Autodesk Fusion 360 part; units mm, degrees
sketch "Sketch5" plane through (0, 0, 4) normal (0, 0, 1) x (-1, 0, 0)
  arc A0 (84, -50) -> (88, -46) centre (84, -46) ccw
  line L0 (88, -46) -> (88, 46)
  arc A1 (88, 46) -> (84, 50) centre (84, 46) ccw
  line L1 (84, 50) -> (-84, 50)
  arc A2 (-84, 50) -> (-88, 46) centre (-84, 46) ccw
  line L2 (-88, 46) -> (-88, -46)
  arc A3 (-88, -46) -> (-84, -50) centre (-84, -46) ccw
  line L3 (-84, -50) -> (84, -50)
  circle A4 centre (69, -43.25) radius 1.425
  circle A5 centre (-69, -43.25) radius 7.5
  circle A6 centre (69, 43.25) radius 7.5
  circle A7 centre (-69, 43.25) radius 7.5
  circle A8 centre (69, -43.25) radius 3.5
  circle A9 centre (-69, -43.25) radius 2.5
  circle A10 centre (-69, 43.25) radius 2.5
  circle A11 centre (69, 43.25) radius 2.5
  line L4 (69, -43.25) -> (-69, -43.25) construction
  line L5 (69, -43.25) -> (69, 43.25) construction
  line L6 (85, -50) -> (85, -42.0241)
  line L7 (85, -42.0241) -> (85, 50) construction
  line L8 (-85, -50) -> (-85, 50) construction
  line L9 (0, -50) -> (0, 50) construction
  circle A12 centre (85, -35) radius 2.25
  circle A13 centre (85, 35) radius 1.425
  circle A14 centre (-85, -35) radius 1.425
  circle A15 centre (-85, 35) radius 1.425
  line L10 (88, 0) -> (-88, 0) construction
  line L11 (85, -35) -> (-85, -35) construction
  line L12 (85, 35) -> (-85, 35) construction
  line L13 (85, -32.75) -> (80, -32.75)
  arc A16 (80, -32.75) -> (80, -37.25) centre (80, -35) ccw
  line L14 (80, -37.25) -> (85, -37.25)
  arc A17 (85, -37.25) -> (85, -32.75) centre (85, -35) ccw
  line L15 (85, -35) -> (80, -35) construction
  line L16 (85, 37.25) -> (80, 37.25)
  arc A18 (80, 37.25) -> (80, 32.75) centre (80, 35) ccw
  line L17 (80, 32.75) -> (85, 32.75)
  arc A19 (85, 32.75) -> (85, 37.25) centre (85, 35) ccw
  line L18 (85, 35) -> (80, 35) construction
  line L19 (-85, -37.25) -> (-80, -37.25)
  arc A20 (-80, -37.25) -> (-80, -32.75) centre (-80, -35) ccw
  line L20 (-80, -32.75) -> (-85, -32.75)
  arc A21 (-85, -32.75) -> (-85, -37.25) centre (-85, -35) ccw
  line L21 (-85, -35) -> (-80, -35) construction
  line L22 (-85, 32.75) -> (-80, 32.75)
  arc A22 (-80, 32.75) -> (-80, 37.25) centre (-80, 35) ccw
  line L23 (-80, 37.25) -> (-85, 37.25)
  arc A23 (-85, 37.25) -> (-85, 32.75) centre (-85, 35) ccw
  line L24 (-85, 35) -> (-80, 35) construction
  point P0 (0, -43.25)
  point P1 (69, 0)
  dimension "d1" = 2.85
  dimension "d2" = 15
  dimension "d3" = 15
  dimension "d4" = 15
  dimension "d5" = 7
  dimension "d6" = 5
  dimension "d7" = 5
  dimension "d8" = 5
  dimension "d9" = 138
  dimension "d10" = 86.5
  dimension "d11" = 4.5
  dimension "d12" = 2.85
  dimension "d13" = 2.85
  dimension "d14" = 2.85
  dimension "d15" = 70
  dimension "d16" = 15
  dimension "d17" = 170
  dimension "d18" = 4.5
  dimension "d19" = 4.5
  dimension "d20" = 5
  dimension "d21" = 4.5
  dimension "d22" = 5
  dimension "d23" = 4.5
sketch "Sketch6" plane through (0, 0, 4) normal (0, 0, 1) x (-1, 0, 0)
  circle A0 centre (85, 35) radius 2.25
  circle A1 centre (-85, 35) radius 2.25
  circle A2 centre (85, -35) radius 2.25
  circle A3 centre (-85, -35) radius 2.25
  arc A4 (-88, -46) -> (-84, -50) centre (-84, -46) ccw
  line L0 (-84, -50) -> (84, -50)
  arc A5 (84, -50) -> (88, -46) centre (84, -46) ccw
  line L1 (88, -46) -> (88, 46)
  arc A6 (88, 46) -> (84, 50) centre (84, 46) ccw
  line L2 (84, 50) -> (-84, 50)
  arc A7 (-84, 50) -> (-88, 46) centre (-84, 46) ccw
  line L3 (-88, 46) -> (-88, -46)
  line L4 (32.925, -38.05) -> (-68.925, -38.05) construction
  line L5 (-68.925, -38.05) -> (-68.925, 38.05) construction
  line L6 (-68.925, 38.05) -> (32.925, 38.05) construction
  line L7 (32.925, 38.05) -> (32.925, -38.05) construction
  circle A8 centre (32.925, -38.05) radius 1.425
  circle A9 centre (32.925, -38.05) radius 3
  circle A10 centre (-68.925, -38.05) radius 1.425
  circle A11 centre (-68.925, -38.05) radius 3
  circle A12 centre (32.925, 38.05) radius 1.425
  circle A13 centre (32.925, 38.05) radius 3
  circle A14 centre (-68.925, 38.05) radius 1.425
  circle A15 centre (-68.925, 38.05) radius 3
  line L8 (22.8962, -40.5575) -> (-22.2991, -40.5575) construction
  line L9 (-22.2991, -40.5575) -> (-22.2991, -50.5575) construction
  line L10 (-22.2991, -50.5575) -> (22.8962, -50.5575) construction
  line L11 (22.8962, -50.5575) -> (22.8962, -40.5575) construction
  line L12 (32.925, -38.05) -> (-68.925, 38.05) construction
  line L13 (-68.925, -38.05) -> (32.925, 38.05) construction
  line L14 (28.925, -30.0681) -> (28.925, 30.0681)
  line L15 (28.925, 30.0681) -> (-11.3172, 0)
  line L16 (-11.3172, 0) -> (28.925, -30.0681)
  line L17 (20.8887, -34.05) -> (-18, -4.9932)
  line L18 (-18, -4.9932) -> (-56.8887, -34.05)
  line L19 (-56.8887, -34.05) -> (20.8887, -34.05)
  line L20 (-64.925, -30.0681) -> (-24.6828, 0)
  line L21 (-24.6828, 0) -> (-64.925, 30.0681)
  line L22 (-64.925, 30.0681) -> (-64.925, -30.0681)
  line L23 (-18, 4.9932) -> (20.8887, 34.05)
  line L24 (20.8887, 34.05) -> (-56.8887, 34.05)
  line L25 (-56.8887, 34.05) -> (-18, 4.9932)
  point P0 (32.925, 0)
  point P1 (0, -38.05)
  point P2 (0, -50)
  point P3 (-18, -38.05)
  dimension "d24" = 101.85
  dimension "d25" = 76.1
  dimension "d26" = 2.85
  dimension "d27" = 2.85
  dimension "d28" = 2.85
  dimension "d29" = 2.85
  dimension "d30" = 6
  dimension "d31" = 6
  dimension "d32" = 6
  dimension "d33" = 6
  dimension "d34" = 4
  dimension "d35" = 4
  dimension "d36" = 4
  dimension "d37" = 4
  dimension "d38" = 4
  dimension "d39" = 4
  dimension "d40" = 4
  dimension "d41" = 4
  dimension "d42" = 70
  dimension "d43" = 88
sketch "Sketch1" plane through (0, 0, 0) normal (0, 0, 1) x (1, 0, 0)
  line L0 (-88, 50) -> (88, 50)
  line L1 (88, 50) -> (88, -50)
  line L2 (88, -50) -> (-88, -50)
  line L3 (-88, -50) -> (-88, 50)
  point P0 (0, 50)
  point P1 (-88, 0)
  dimension "d57" = 176
  dimension "d58" = 100
extrude "Extrude1" add sketch "Sketch1" along normal blind 4
fillet "Fillet2" radius 4 4 edges at (-88, -50, 2) (-88, 50, 2) (88, -50, 2) (88, 50, 2)
extrude "Extrude5" cut sketch "Sketch5" against normal through all contours A12 A17 | A13 | A14 | A15
sketch "Sketch3" plane through (0, 0, 0) normal (0, 0, -1) x (1, 0, 0)
  arc A0 (84, -50) -> (88, -46) centre (84, -46) ccw
  line L0 (88, -46) -> (88, 46)
  arc A1 (88, 46) -> (84, 50) centre (84, 46) ccw
  line L1 (84, 50) -> (-84, 50)
  arc A2 (-84, 50) -> (-88, 46) centre (-84, 46) ccw
  line L2 (-88, 46) -> (-88, -46)
  arc A3 (-88, -46) -> (-84, -50) centre (-84, -46) ccw
  line L3 (-84, -50) -> (84, -50)
  line L4 (-35, -19) -> (35, -19)
  line L5 (35, -19) -> (35, -31)
  line L6 (35, -31) -> (-35, -31)
  line L7 (-35, -31) -> (-35, -19)
  circle A4 centre (-85, 35) radius 1.425
  circle A5 centre (85, 35) radius 1.425
  circle A6 centre (-85, -35) radius 2.25
  circle A7 centre (85, -35) radius 1.425
  line L8 (85, -35) -> (-85, -35) construction
  point P0 (0, -19)
  point P1 (35, -25)
  dimension "d86" = 70
  dimension "d87" = 12
  dimension "d129" = 4
extrude "Extrude4" cut sketch "Sketch3" against normal blind 3 contours L4 L5 L6 L7
fillet "Fillet3" radius 3 4 edges at (-35, 19, 1.5) (-35, 31, 1.5) (35, 31, 1.5) (35, 19, 1.5)
sketch "Sketch4" plane through (1.194, -0.2204, 4) normal (0, 0, 1) x (-1, 0, 0)
  circle A0 centre (86.194, 34.7796) radius 1.425
  circle A1 centre (-83.806, 34.7796) radius 1.425
  circle A2 centre (86.194, -35.2204) radius 2.25
  circle A3 centre (-83.806, -35.2204) radius 1.425
  arc A4 (-86.806, -46.2204) -> (-82.806, -50.2204) centre (-82.806, -46.2204) ccw
  line L0 (-82.806, -50.2204) -> (85.194, -50.2204)
  arc A5 (85.194, -50.2204) -> (89.194, -46.2204) centre (85.194, -46.2204) ccw
  line L1 (89.194, -46.2204) -> (89.194, 45.7796)
  arc A6 (89.194, 45.7796) -> (85.194, 49.7796) centre (85.194, 45.7796) ccw
  line L2 (85.194, 49.7796) -> (-82.806, 49.7796)
  arc A7 (-82.806, 49.7796) -> (-86.806, 45.7796) centre (-82.806, 45.7796) ccw
  line L3 (-86.806, 45.7796) -> (-86.806, -46.2204)
  line L4 (86.194, -32.9704) -> (81.194, -32.9704)
  arc A8 (81.194, -32.9704) -> (81.194, -37.4704) centre (81.194, -35.2204) ccw
  line L5 (81.194, -37.4704) -> (86.194, -37.4704)
  arc A9 (86.194, -37.4704) -> (86.194, -32.9704) centre (86.194, -35.2204) ccw
  line L6 (86.194, -35.2204) -> (81.194, -35.2204) construction
  line L7 (86.194, 37.0296) -> (81.194, 37.0296)
  arc A10 (81.194, 37.0296) -> (81.194, 32.5296) centre (81.194, 34.7796) ccw
  line L8 (81.194, 32.5296) -> (86.194, 32.5296)
  arc A11 (86.194, 32.5296) -> (86.194, 37.0296) centre (86.194, 34.7796) ccw
  line L9 (86.194, 34.7796) -> (81.194, 34.7796) construction
  line L10 (-83.806, -37.4704) -> (-78.806, -37.4704)
  arc A12 (-78.806, -37.4704) -> (-78.806, -32.9704) centre (-78.806, -35.2204) ccw
  line L11 (-78.806, -32.9704) -> (-83.806, -32.9704)
  arc A13 (-83.806, -32.9704) -> (-83.806, -37.4704) centre (-83.806, -35.2204) ccw
  line L12 (-83.806, -35.2204) -> (-78.806, -35.2204) construction
  line L13 (-83.806, 32.5296) -> (-78.806, 32.5296)
  arc A14 (-78.806, 32.5296) -> (-78.806, 37.0296) centre (-78.806, 34.7796) ccw
  line L14 (-78.806, 37.0296) -> (-83.806, 37.0296)
  arc A15 (-83.806, 37.0296) -> (-83.806, 32.5296) centre (-83.806, 34.7796) ccw
  line L15 (-83.806, 34.7796) -> (-78.806, 34.7796) construction
  dimension "d292" = 4.5
  dimension "d293" = 170
  dimension "d294" = 5
  dimension "d295" = 4.5
  dimension "d296" = 4.5
  dimension "d297" = 4.5
  dimension "d298" = 5
extrude "Extrude7" cut sketch "Sketch4" against normal blind 4 contours A2 L4 A8 L5 | L7 A10 L8 A11 | L10 A12 L11 A13 | L13 A14 L14 A15
extrude "Extrude6" cut sketch "Sketch6" against normal through all contours L14 L15 L16 | L17 L18 L19 | L20 L21 L22 | L23 L24 L25
fillet "Fillet4" radius 4 2 edges at (11.3172, 0, 2) (-28.925, -30.0681, 2)
fillet "Fillet5" radius 4 1 edges at (56.8887, -34.05, 2)
equation "d2 = d16"
equation "d3 = d16"
equation "d4 = d16"
equation "d6 = d20"
equation "d7 = d20"
equation "d8 = d20"
equation "d12 = d29"
equation "d13 = d29"
equation "d14 = d29"
Design review of the part built by this model. Coordinates are the model's own, in mm. A direction names the side the tool comes from. Coordinates: 2 decimals unless noted, no trailing zeros. Order: outer loops, then holes, each group sorted by start corner. A loop starts at its lowest first (then second) coordinate and runs counter-clockwise, first axis right, second up.
1) For faces 4 (the cylindrical face through (77.75, -34.95, 2.03)), 5 (the flat face through (-1, -10, 4)), 6 (the flat face through (-22, 26, 3)), list the 3-axis set-ups (+Z, -Z, +X, -X, +Y, -Y) from which the entire face can be reached by the end or side of a thin tool; tool diameter is ignored.
2) Take a section at C-C, the plane z = 0.95. State how many separate pieces and enclosed holes the cut face has, and give its area (3 significant figures).
3) Take a section at A-A, the plane y = 8. Give the boundary of the cut face in (x, z) (3 decimals).
4) Clearance check with a flat-ended pin moving along its axis: pin 1 (9.5 mm diameter, centred on x = -13, y = 25.5, fed in from -Z). State where the tip first meets the part, or that it passes through.
5) Take a section at B-B, the plane x = -24.5. Give the boundary of the cut face in (y, z).
6) Take a section at D-D, the plane y = 26. Give the boundary of the cut face in (x, z) (3 decimals).
7) Wall thickness on line 1 along X through (y, z) = (34, 3.25); line 2 along Y through (x, z) = (20, 1.05); line 3 along Y through (x, z) = (55, 3): over which ranges is each line inside the solid? List them lowest first.
8) Mouldability with a two-part tool opening along Y and no side actions: class faces 1 (the flat face through (82, 32.75, 2)), 2 (the cylindrical face through (-86.797, 48.859, 2.028)), 3 (the flat face through (-88, -1, 2)) as +Y half, -Y half, draft (parallel to the pull), parting line (faces both ways), or undercut.
Returned:
1. face 4: +Z, -Z
1. face 5: +Z, +X, -X, +Y, -Y
1. face 6: -Z
2. separate pieces: 1
2. enclosed holes: 7
2. area: 12,600 mm2
3. outline: (-88, 0) - (-28.925, 0) - (-28.925, 4) - (-88, 4) - close; (0.61, 0) - (13.976, 0) - (13.976, 4) - (0.61, 4) - close; (22.024, 0) - (35.39, 0) - (35.39, 4) - (22.024, 4) - close; (64.925, 0) - (88, 0) - (88, 4) - (64.925, 4) - close
4. pin 1: stops at z = 3
5. outline: (-50, 0) - (-26.06, 0) - (-26.06, 4) - (-50, 4) - close; (26.76, 3) - (31, 3) - (31, 0) - (50, 0) - (50, 4) - (26.76, 4) - close
6. outline: (-88, 0) - (-35, 0) - (-35, 3) - (-28.925, 3) - (-28.925, 4) - (-88, 4) - close; (-23.48, 3) - (-10.115, 3) - (-10.115, 4) - (-23.48, 4) - close; (46.115, 0) - (59.48, 0) - (59.48, 4) - (46.115, 4) - close; (64.925, 0) - (88, 0) - (88, 4) - (64.925, 4) - close
7. line 1: x = -88 to -87.02, -77.98 to -20.82, 56.82 to 77.98, 87.02 to 88
7. line 2: y = -50 to -34.05, -6.49 to 6.49, 34.05 to 50
7. line 3: y = -50 to -22.65, 22.65 to 32.64, 34.05 to 50
8. face 1: undercut
8. face 2: +Y half
8. face 3: draft
